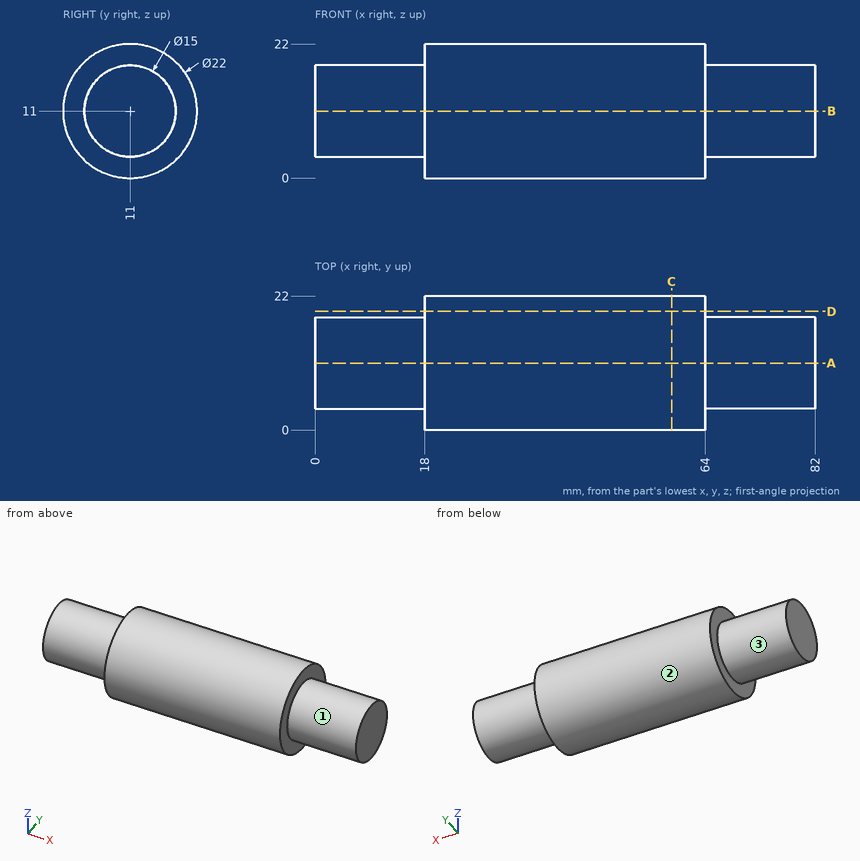
Can you work these out from the drawing? Everything is in mm from the part's minimum corner. A direction names the side the tool comes from. Round coordinates to 2 decimals unless told otherwise and drop trailing zeros. Order: outer loops, then holes, each group sorted by start corner. A loop starts at its lowest first (then second) coordinate and runs counter-clockwise, first axis right, second up. Notation, with made-up numbers: (57, 50) -> (114, 50) arc R23 cw to (114, 59) -> close; hole circle Ø11 at (-12.5, 15.5). An arc over 180 degrees is marked (long way). Use CSV: the item, a comma, the result in double quotes.
1. I want a section at D-D on y = 19.5. List the corners of the cut face in (x, z) for me, and give its area (3 significant figures).
Recorded:
outline,"(18, 4.02) -> (64, 4.02) -> (64, 17.98) -> (18, 17.98) -> close"
area,"642 mm2"
2. I want a section at A-A on y = 11. List the corners of the cut face in (x, z) for me.
Recorded:
outline,"(0, 3.5) -> (18, 3.5) -> (18, 0) -> (64, 0) -> (64, 3.5) -> (82, 3.5) -> (82, 18.5) -> (64, 18.5) -> (64, 22) -> (18, 22) -> (18, 18.5) -> (0, 18.5) -> close"
3. I'm going to push flat-ended pins straight in: P1, Ø3, axis at x = 46.5, z = 8, coming from the -Y side; P2, Ø10, axis at x = 36, y = 18, coming from the -Z side; P3, Ø1, axis at x = 58.5, y = 13, coming from the +Z side. Where does each tip first touch, or does it pass through?
Recorded:
P1,"stops at y = 0.1"
P2,"stops at z = 0.18"
P3,"stops at z = 21.9"
4. I need wall thicknesses on line 1 along X through (y, z) = (10.5, 1.75); line 2 along Y through (x, z) = (39.5, 6.75); line 3 along Y through (x, z) = (58, 7.75). Which ranges of each line are inside material? Lowest first, please.
Recorded:
line 1,"x = 18 to 64"
line 2,"y = 0.85 to 21.15"
line 3,"y = 0.49 to 21.51"
5. Which directions (+Z, -Z, +X, -X, +Y, -Y) give clear straight access to the entire face, cutting with the end or side of a thin tool? Please do the marked faces 1, 2 and 3.
Recorded:
face 1,"+X"
face 2,"+X, -X"
face 3,"-X"
6. I want a section at C-C on x = 58.5. List the corners of the cut face in (y, z) for me, and give its area (3 significant figures).
Recorded:
outline,"circle Ø22 at (11, 11)"
area,"380 mm2"
